Can you work these out from the model? Positions are in its coordinate system, mm. Face numbers are marked on the shaded views. A direction names the side the tool comes from. Round coordinates to 2 decimals unless told otherwise and drop trailing zeros. Loops run counter-clockwise (first coordinate to the right, second up) from the corner with the lowest first, then second, coordinate; pieces in that order, holes last.
```python
from build123d import *

# Parameters (mm, degrees)
SKETCH2_W           = 17
SKETCH2_H           = 13.5
SKETCH2_W_2         = 7
SKETCH2_H_2         = 3.5
BOSS_EXTRUDE1_DEPTH = 15
SKETCH3_R           = 2.15
CUT_EXTRUDE1_DEPTH  = 15
BOSS_EXTRUDE2_START = 2
SKETCH4_R           = 3.15
SKETCH4_R_2         = 2.15
BOSS_EXTRUDE2_DEPTH = 2


with BuildPart() as part:
    # Sketch2 → Boss-Extrude1 (new body)
    with BuildSketch(Plane.XY):
        Rectangle(SKETCH2_W, SKETCH2_H)
        Rectangle(SKETCH2_W_2, SKETCH2_H_2, mode=Mode.SUBTRACT)
    extrude(amount=BOSS_EXTRUDE1_DEPTH)

    # Sketch3 → Cut-Extrude1 (cut)
    with BuildSketch(Plane(origin=(0, 6.75, 0), x_dir=(1, 0, 0), z_dir=(0, 1, 0))):
        with Locations(Location((0, -7.5, 0), (0, 0, 270))):
            Circle(SKETCH3_R)
    extrude(amount=-CUT_EXTRUDE1_DEPTH, mode=Mode.SUBTRACT)

    # Sketch4 → Boss-Extrude2 (add)
    with BuildSketch(Plane(origin=(0, 6.75, 0), x_dir=(1, 0, 0), z_dir=(0, 1, 0)).offset(BOSS_EXTRUDE2_START)):
        with Locations(Location((0, -7.5, 0), (0, 0, 90))):
            Circle(SKETCH4_R)
        with Locations(Location((0, -7.5, 0), (0, 0, 270))):
            Circle(SKETCH4_R_2, mode=Mode.SUBTRACT)
    extrude(amount=-BOSS_EXTRUDE2_DEPTH)


solid = part.part
```
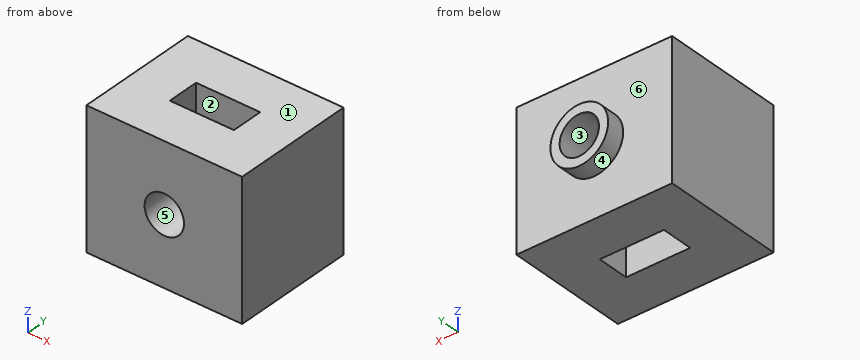
(1) If I drill on line 1 (X direction, y = -4.4, z = 7.5); line 2 (X direction, y = 0, z = 10.25); line 3 (Y direction, x = -5, z = 13), over which ranges is the centre line in solid material (lowest first)?
(2) Suppose I cut it at C-C (y = 4.75). Write out the boundary of the cut face in (x, z).
(3) We'd pull the mould along Z, two halves only. Please class the marked faces 3, 4, 5 and 6: released by +Z, released by -Z, zero draft, split by the parting line, or undercut.
(4) Which directions (+Z, -Z, +X, -X, +Y, -Y) give clear straight access to the entire face, cutting with the end or side of a thin tool? Please do the marked faces 1 and 2.
(5) Suppose I cut it at A-A (x = 0). Write out the boundary of the cut face in (y, z).
(6) Suppose I cut it at D-D (z = 7.5). Write out the boundary of the cut face in (x, y), then the cut area to 3 significant figures.
(7) Suppose I cut it at B-B (z = 12.75). Write out the boundary of the cut face in (x, y).
Check result:
1. line 1: x = -8.5 to -2.15, 2.15 to 8.5
1. line 2: x = -8.5 to -3.5, 3.5 to 8.5
1. line 3: y = -6.75 to 6.75
2. outline: (-8.5, 0) - (8.5, 0) - (8.5, 15) - (-8.5, 15) - close; hole circle Ø4.3 at (0, 7.5)
3. face 3: undercut
3. face 4: split by the parting line
3. face 5: undercut
3. face 6: zero draft
4. face 1: +Z, +X, -X, +Y, -Y
4. face 2: +Z, -Z
5. outline: (-6.75, 0) - (-1.75, 0) - (-1.75, 5.35) - (-6.75, 5.35) - close; (-6.75, 9.65) - (-1.75, 9.65) - (-1.75, 15) - (-6.75, 15) - close; (1.75, 0) - (6.75, 0) - (6.75, 4.35) - (8.75, 4.35) - (8.75, 5.35) - (1.75, 5.35) - close; (1.75, 9.65) - (8.75, 9.65) - (8.75, 10.65) - (6.75, 10.65) - (6.75, 15) - (1.75, 15) - close
6. outline: (-8.5, -6.75) - (-2.15, -6.75) - (-2.15, -1.75) - (-3.5, -1.75) - (-3.5, 1.75) - (-2.15, 1.75) - (-2.15, 8.75) - (-3.15, 8.75) - (-3.15, 6.75) - (-8.5, 6.75) - close; (2.15, -6.75) - (8.5, -6.75) - (8.5, 6.75) - (3.15, 6.75) - (3.15, 8.75) - (2.15, 8.75) - (2.15, 1.75) - (3.5, 1.75) - (3.5, -1.75) - (2.15, -1.75) - close
6. area: 166 mm2
7. outline: (-8.5, -6.75) - (8.5, -6.75) - (8.5, 6.75) - (-8.5, 6.75) - close; hole (-3.5, -1.75) - (3.5, -1.75) - (3.5, 1.75) - (-3.5, 1.75) - close
